from build123d import *

# Parameters (mm, degrees)
SKETCH1_R           = 5
SKETCH1_R_2         = 1.5
BOSS_EXTRUDE1_DEPTH = 2.5
SKETCH2_W           = 1
SKETCH2_H           = 4


with BuildPart() as part:
    # Sketch1 → Boss-Extrude1 (new, symmetric)
    with BuildSketch(Plane(origin=(0, 0, 0), x_dir=(1, 0, 0), z_dir=(0, 1, 0))):
        with Locations(Location((0, 0, 0), (0, 0, 270))):
            Circle(SKETCH1_R)
        with Locations(Location((0, 0, 0), (0, 0, 270))):
            Circle(SKETCH1_R_2, mode=Mode.SUBTRACT)
    extrude(amount=BOSS_EXTRUDE1_DEPTH, both=True)

    # Sketch2 → Cut-Revolve1 (revolve, cut)
    with BuildSketch(Plane(origin=(0, 0, 0), x_dir=(0, 0, -1), z_dir=(1, 0, 0)), mode=Mode.PRIVATE) as cut_revolve1_sk:
        with Locations((-4.5, 0)):
            Rectangle(SKETCH2_W, SKETCH2_H)
    revolve(cut_revolve1_sk.sketch.rotate(Axis((0, 0, 0), (0, 1, 0)), 180), axis=Axis((0, 0, 0), (0, 1, 0)), mode=Mode.SUBTRACT)


solid = part.part
CAD build for the part. Positions are in the model's coordinates, mm. Coordinates: 2 decimals unless noted, no trailing zeros. Write each loop counter-clockwise with the first axis right and the second up, starting at its lowest first coordinate (ties: lowest second). Pieces come first, ordered by that corner, then holes. Notation, with made-up numbers: M -19.5,33 L 12.5,33 A18 ccw 12.5,50 Z; hole C 43,64.5 d3. An arc over 180 degrees is marked long. Answer as a JSON object with one key per item and string values. Group by question number.
1) Wall check: line 1 (X direction, y = -0.5, z = 0); line 2 (Y direction, x = 3.5, z = -2.75); line 3 (X direction, y = 0.4, z = -0.75). Give the ranges that are in metal, low to high. Write a range as from..to.
2) Saw through at B-B (x = 0). Write the cut outline in (y, z).
3) Saw through at D-D (z = 2.75). Write the cut outline in (x, y).
4) Saw through at A-A (z = 0). Write the cut outline in (x, y), plus the area to 3 significant figures.
5) Saw through at C-C (y = -0.75). Write the cut outline in (x, z), plus the area to 3 significant figures.
6) Pin check, flat tips, straight feed: pin 1 Ø5 at (x, z) = (-1, 0.5) entering from +Y; pin 2 Ø1.5 at (y, z) = (2, 1) entering from +X; pin 3 Ø2.5 at (x, z) = (0, 0) entering from +Y. Stop position of each tip, or through.
7) Mould opens along X. For faces 1 (the face through (0.45, -0.04, 1.43)), 2 (the face through (3.905, 0.028, 0.867)), 3 (the face through (1.2, -2.5, -1.2)) say: +X half, -X half, draft (parallel to the pull), parting line (faces both ways), or undercut.
Values follow:
{
 "1": {"line 1": "x = -4..-1.5, 1.5..4", "line 2": "y = -2.5..-2, 2..2.5", "line 3": "x = -3.93..-1.3, 1.3..3.93"},
 "2": {"outline": "M -2.5,-5 L -2,-5 L -2,-4 L 2,-4 L 2,-5 L 2.5,-5 L 2.5,-1.5 L -2.5,-1.5 Z; M -2.5,1.5 L 2.5,1.5 L 2.5,5 L 2,5 L 2,4 L -2,4 L -2,5 L -2.5,5 Z"},
 "3": {"outline": "M -4.18,-2.5 L 4.18,-2.5 L 4.18,-2 L 2.9,-2 L 2.9,2 L 4.18,2 L 4.18,2.5 L -4.18,2.5 L -4.18,2 L -2.9,2 L -2.9,-2 L -4.18,-2 Z"},
 "4": {"outline": "M -5,-2.5 L -1.5,-2.5 L -1.5,2.5 L -5,2.5 L -5,2 L -4,2 L -4,-2 L -5,-2 Z; M 1.5,-2.5 L 5,-2.5 L 5,-2 L 4,-2 L 4,2 L 5,2 L 5,2.5 L 1.5,2.5 Z", "area": "27.0 mm2"},
 "5": {"outline": "C 0,0 d8; hole C 0,0 d3", "area": "43.2 mm2"},
 "6": {"pin 1": "stops at y = 2.5", "pin 2": "stops at x = 4.99", "pin 3": "passes through"},
 "7": {"face 1": "undercut", "face 2": "parting line", "face 3": "draft"}
}
